```python
from build123d import *


with BuildPart() as part:
    # Sketch1 → Revolve1 (revolve)
    with BuildSketch(Plane.XY):
        Polygon((0, 7), (-0.5, 7), (-0.5, 8), (-3, 8), (-3, 9.5), (-2, 10.5), (0, 10.5), align=None)
    revolve1 = revolve(axis=Axis((0, 0, 0), (-1, 0, 0)))

    # Mirror1: Revolve1 across plane
    add(revolve1.mirror(Plane(origin=(0, 10.5, 0), x_dir=(0, 0, 1), z_dir=(1, 0, 0))))


solid = part.part
```
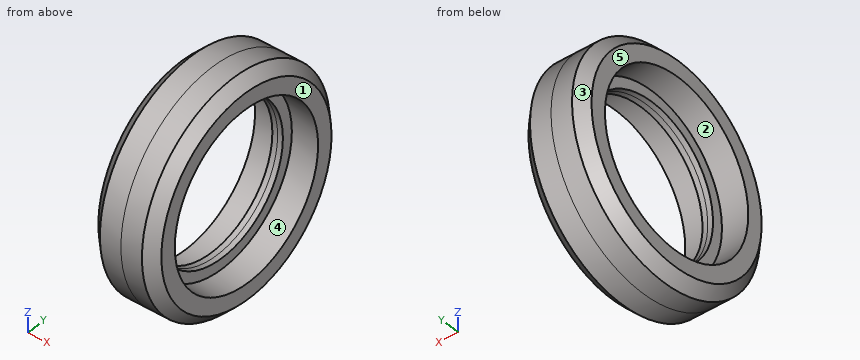
CAD build for the part. Positions are in the model's coordinates, mm. Face numbers are marked on the shaded views. A direction names the side the tool comes from. Coordinates: 2 decimals unless noted, no trailing zeros. Order: outer loops, then holes, each group sorted by start corner. A loop starts at its lowest first (then second) coordinate and runs counter-clockwise, first axis right, second up.
(1) Saw through at A-A, the plane z = 0. Write the cut outline in (x, y), and give its area (3 significant figures).
Solution:
outline: (-3, -9.5) - (-2, -10.5) - (2, -10.5) - (3, -9.5) - (3, -8) - (0.5, -8) - (0.5, -7) - (-0.5, -7) - (-0.5, -8) - (-3, -8) - close; (-3, 8) - (-0.5, 8) - (-0.5, 7) - (0.5, 7) - (0.5, 8) - (3, 8) - (3, 9.5) - (2, 10.5) - (-2, 10.5) - (-3, 9.5) - close
area: 30.0 mm2
(2) Pin check, flat tips, straight feed: pin 1 Ø5 at (y, z) = (-2, 5) entering from +X; pin 2 Ø1 at (x, y) = (0.5, -7.5) entering from -Z; pin 3 Ø3 at (x, y) = (-2.5, -7.5) entering from +Z. Stop position of each tip, or through.
Solution:
pin 1: stops at x = 0.5
pin 2: stops at z = -7.83
pin 3: stops at z = 8.56
(3) Drill centre lines: L1, parallel to Z at x = -0.05, y = 0; L2, parallel to Z at x = 1.8, y = 0. Where is each one in solid material? Low to high.
Solution:
L1: z = -10.5 to -7, 7 to 10.5
L2: z = -10.5 to -8, 8 to 10.5
(4) Which spindle directions (+Z, -Z, +X, -X, +Y, -Y) get a long thin tool onto all of the face, cutting with end or side? Do the marked faces 4 and 5. Say none if no direction does.
Solution:
face 4: +X
face 5: +Z, -Z, -X, +Y, -Y
(5) Mould opens along Y. For the marked faces 1, 2 and 3 say: released by +Y, released by -Y, zero draft, split by the parting line, or undercut.
Solution:
face 1: zero draft
face 2: undercut
face 3: split by the parting line
(6) Saw through at C-C, the plane x = 1.75. Write the cut outline in (y, z).
Solution:
outline: circle Ø21 at (0, 0); hole circle Ø16 at (0, 0)
